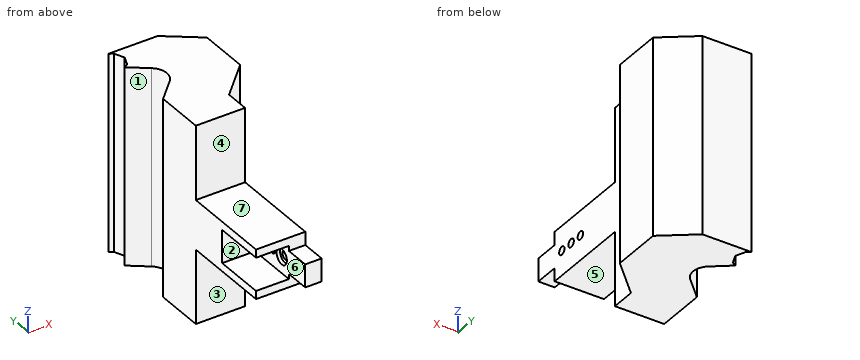
Autodesk Inventor part; units mm, degrees
ref_plane "Work Plane1" through (0, 0, -15) normal (0, 0, 1) x (1, 0, 0)
ref_plane "YZ Plane" through (0, 0, 0) normal (1, 0, 0) x (0, 1, 0)
ref_plane "XZ Plane" through (0, 0, 0) normal (0, 1, 0) x (-1, 0, 0)
sketch "Sketch1" plane through (0, 0, 0) normal (0, 0, 1) x (1, 0, 0)
  line L0 (0, 0) -> (25, 0)
  line L1 (25, 0) -> (25, 40)
  line L2 (25, 40) -> (0, 40)
  line L3 (0, 40) -> (0, 0)
  dimension "d1" = 25
  dimension "d2" = 40
  dimension "d3" = 25
extrude "Extrusion1" add sketch "Sketch1" against normal blind 30
sketch "Sketch2" plane through (25, 0, 0) normal (1, 0, 0) x (0, 0, -1)
  line L0 (0, 0) -> (30, 0)
  circle A0 centre (15, 6.56) radius 2.46
extrude "Extrusion2" cut sketch "Sketch2" against normal blind 30
sketch "Sketch3" plane through (0, 0, 0) normal (-1, 0, 0) x (0, 0, 1)
  line L0 (0, 0) -> (-30, 0)
  line L1 (-25.05, 0) -> (-4.95, 0)
  line L2 (-4.95, 0) -> (-4.95, 33.12)
  line L3 (-4.95, 33.12) -> (-25.05, 33.12)
  line L4 (-25.05, 33.12) -> (-25.05, 0)
  dimension "d11" = 20.1
extrude "Extrusion3" cut sketch "Sketch3" against normal blind 20
sketch "Sketch4" plane through (0, 0, 0) normal (0, -1, 0) x (1, 0, 0)
  line L0 (20, -4.95) -> (20, -25.05)
  line L1 (20, -15) -> (25, -15)
  line L2 (25, 0) -> (25, -30)
  line L3 (20, -8.025) -> (25, -8.025)
  line L4 (25, -8.025) -> (25, -21.975)
  line L5 (25, -21.975) -> (20, -21.975)
  line L6 (20, -21.975) -> (20, -8.025)
  line L7 (20, -8.025) -> (25, -21.975) construction
  line L8 (25, -8.025) -> (20, -21.975) construction
  line L9 (25, -12.54) -> (25, -17.46)
  point P0 (0, 0)
  point P1 (22.5, -15)
  dimension "d14" = 13.95
extrude "Extrusion4" add sketch "Sketch4" along normal blind 15
sketch "Sketch5" plane through (20, 0, 0) normal (-1, 0, 0) x (0, 0, 1)
  circle A0 centre (-15, 6.56) radius 2.46
  circle A1 centre (-15, 6.56) radius 4.7025
  circle A2 centre (-15, 6.56) radius 2.46
  circle A3 centre (-15, 6.56) radius 2.46
  point P0 (0, 0)
  dimension "d17" = 9.405
extrude "Extrusion5" cut sketch "Sketch5" against normal blind 2.1
sketch "Sketch6" plane through (25, 0, 0) normal (1, 0, 0) x (0, 0, -1)
  circle A0 centre (15, 6.56) radius 4.7025
  line L0 (15, 6.56) -> (15, 23.56)
  circle A1 centre (15, 23.56) radius 2.46
  point P0 (0, 0)
  dimension "d20" = 17
  dimension "d21" = 4.92
extrude "Extrusion6" cut sketch "Sketch6" against normal blind 10 contours A1
sketch "Sketch7" plane through (20, 0, 0) normal (-1, 0, 0) x (0, 0, 1)
  circle A0 centre (-15, 23.56) radius 2.46
  circle A1 centre (-15, 23.56) radius 4.7025
  point P0 (0, 0)
  dimension "d24" = 9.405
extrude "Extrusion7" cut sketch "Sketch7" against normal blind 2.1
sketch "Sketch9" plane through (25, 0, 0) normal (1, 0, 0) x (0, 0, -1)
  circle A0 centre (15, 6.56) radius 2.46
  circle A1 centre (15, 6.56) radius 2.46
  circle A2 centre (15, 23.56) radius 2.46
  circle A3 centre (15, 23.56) radius 2.46
  line L0 (30, 40) -> (30, 0)
  line L1 (30, 0) -> (30, 40)
  line L2 (30, 40) -> (0, 40)
  line L3 (0, 40) -> (0, 0)
  line L4 (0, 0) -> (8.025, 0)
  line L5 (21.975, 0) -> (21.975, -15)
  line L6 (21.975, -15) -> (8.025, -15)
  line L7 (8.025, -15) -> (8.025, 0)
  line L8 (0, 0) -> (8.025, 0)
  line L9 (21.975, 0) -> (30, 0)
extrude "Extrusion8" add sketch "Sketch9" along normal blind 5
sketch "Sketch10" plane through (0, 40, 0) normal (0, 1, 0) x (1, 0, 0)
  line L0 (0, 30) -> (30, 30)
  line L1 (30, 0) -> (0, 0)
  line L2 (0, 30) -> (30, 30)
  line L3 (30, 30) -> (30, 0)
  line L4 (30, 0) -> (0, 0)
  line L5 (0, 0) -> (0, 30)
extrude "Extrusion9" add sketch "Sketch10" along normal blind 30
sketch "Sketch12" plane through (30, 0, 0) normal (1, 0, 0) x (0, 0, -1)
  circle A0 centre (15, 6.56) radius 2.46
  line L0 (15, 6.56) -> (15, 15.06)
  circle A1 centre (15, 15.06) radius 2.525
  point P0 (0, 0)
  dimension "d31" = 8.5
  dimension "d33" = 5.05
extrude "Extrusion10" cut sketch "Sketch12" against normal blind 30 contours A1
sketch "Sketch15" plane through (0, 0, -25.05) normal (-1, 0, 0) x (0, 0, 1)
  line L0 (0, 33.12) -> (20.1, 33.12)
  line L1 (20.1, 33.12) -> (20.1, 0)
  line L2 (0, 33.12) -> (20.1, 33.12)
  line L3 (20.1, 33.12) -> (20.1, 31.1)
  line L4 (20.1, 31.1) -> (0, 31.1)
  line L5 (0, 31.1) -> (0, 33.12)
  point P0 (25.05, 0)
  dimension "d57" = 2.02
extrude "Extrusion13" add sketch "Sketch15" against normal blind 20
sketch "Sketch17" plane through (0, 0, 0) normal (0, 0, 1) x (1, 0, 0)
  line L0 (0, 70) -> (30, 70)
  line L1 (30, 70) -> (50.0622, 90.0622)
  line L2 (30, 70) -> (80, 70) construction
  line L3 (11.9522, 97.2454) -> (0, 85.2932)
  line L4 (0, 70) -> (0, 85.2932)
  line L5 (0, 70) -> (0, 0)
  line L6 (0, 70) -> (30, 70)
  line L7 (10.923, 112.2849) -> (0, 120.567)
  line L8 (2.5, 134.067) -> (0, 135.567)
  line L9 (2.5, 134.067) -> (5, 128.067)
  line L10 (2.5, 122.067) -> (0, 120.567)
  line L11 (2.5, 122.067) -> (5, 128.067)
  line L12 (50.0622, 105.3553) -> (50.0622, 120.567)
  line L13 (50.0622, 105.3553) -> (50.0622, 90.0622)
  line L14 (0, 135.567) -> (30, 135.567)
  line L15 (30, 135.567) -> (50.0622, 120.567)
  arc A0 (11.9522, 97.2454) -> (10.923, 112.2849) centre (4.8811, 104.3165) ccw
  dimension "d61" = 45
  dimension "d62" = 32.0271
  dimension "d71" = 30
  dimension "d72" = 10
extrude "Extrusion14" add sketch "Sketch17" against normal blind 30
sketch "Sketch19" plane through (0, 0, 0) normal (0, 0, 1) x (1, 0, 0)
  line L0 (30, 0) -> (30, 70)
  line L1 (30, 70) -> (50.0622, 90.0622)
  line L2 (30, 70) -> (50.0622, 90.0622)
  line L3 (50.0622, 120.567) -> (50.0622, 90.0622)
  line L4 (50.0622, 90.0622) -> (50.0622, 120.567)
  line L5 (30, 135.567) -> (50.0622, 120.567)
  line L6 (50.0622, 120.567) -> (30, 135.567)
  line L7 (0, 135.567) -> (30, 135.567)
  line L8 (30, 135.567) -> (0, 135.567)
  line L9 (5, 128.067) -> (2.5, 134.067)
  line L10 (0, 135.567) -> (2.5, 134.067)
  line L11 (2.5, 134.067) -> (5, 128.067)
  line L12 (2.5, 122.067) -> (5, 128.067)
  line L13 (5, 128.067) -> (2.5, 122.067)
  line L14 (0, 120.567) -> (2.5, 122.067)
  line L15 (2.5, 122.067) -> (0, 120.567)
  line L16 (10.923, 112.2849) -> (0, 120.567)
  line L17 (0, 120.567) -> (10.923, 112.2849)
  line L18 (11.9522, 97.2454) -> (0, 85.2932)
  line L19 (11.9522, 97.2454) -> (0, 85.2932)
  line L20 (0, 85.2932) -> (0, 55.2932)
  line L21 (0, 0) -> (0, 85.2932)
  line L22 (0, 55.2932) -> (30, 55.2932)
  line L23 (30, 55.2932) -> (30, 70)
  arc A0 (11.9522, 97.2454) -> (10.923, 112.2849) centre (4.8811, 104.3165) ccw
  dimension "d75" = 30
  dimension "d76" = 30
extrude "Extrusion15" add sketch "Sketch19" along normal blind 45
ref_plane "Work Plane1" through (0, 0, -15) normal (0, 0, 1) x (1, 0, 0)
mirror "Mirror1" about plane through (0, 0, -15) normal (0, 0, 1) of "Extrusion15"
properties part number "rec_c_12mm_x_120mm"
Here's how the part is built. I have some questions about the finished solid (model axes, mm). Face numbers are marked on the shaded views. A direction names the side the tool comes from. Round coordinates to 2 decimals unless told otherwise and drop trailing zeros. Order: outer loops, then holes, each group sorted by start corner. A loop starts at its lowest first (then second) coordinate and runs counter-clockwise, first axis right, second up. Notation, with made-up numbers: (38, -18.5) -> (94, -18.5) arc R21 ccw to (94, 13.5) -> close; hole circle Ø3 at (-35.5, -35). An arc over 180 degrees is marked (long way). Return JSON: item names as keys, results as strings.
Q1. Which directions (+Z, -Z, +X, -X, +Y, -Y) give clear straight access to the entire face, cutting with the end or side of a thin tool? Please do the marked faces 1, 2 and 3.
Filled sheet:
{"face 1": "+Z, -Z, -X", "face 2": "-X, -Y", "face 3": "-Z, +X, -X, -Y"}
Q2. I need wall thicknesses on line 1 along Y through (x, z) = (21.5, -15) (1 decimal); line 2 along Y through (x, z) = (25.25, -15) (3 decimals); line 3 along Z through (x, y) = (11, 8). Which ranges of each line are inside material? Lowest first, please. Write a range as from..to.
Filled sheet:
{"line 1": "y = -15..1.9, 11.3..12.5, 17.6..18.9, 28.3..135.6", "line 2": "y = -15..4.1, 9.02..12.535, 17.585..21.1, 26.02..135.567", "line 3": "z = -30..-25.05, -4.95..0"}
Q3. If we section it at C-C on z = 14: List the corners of the cut face in (x, y) for me.
Filled sheet:
{"outline": "(0, 55.29) -> (30, 55.29) -> (30, 70) -> (50.06, 90.06) -> (50.06, 120.57) -> (30, 135.57) -> (0, 135.57) -> (2.5, 134.07) -> (5, 128.07) -> (2.5, 122.07) -> (0, 120.57) -> (10.92, 112.28) arc R10 cw to (11.95, 97.25) -> (0, 85.29) -> close"}
Q4. If we section it at D-D on x = 8: List the corners of the cut face in (y, z) for me, plus the area to 3 significant figures.
Filled sheet:
{"outline": "(0, -30) -> (55.29, -30) -> (55.29, -75) -> (93.29, -75) -> (93.29, 45) -> (55.29, 45) -> (55.29, 0) -> (0, 0) -> (0, -4.95) -> (31.1, -4.95) -> (31.1, -25.05) -> (0, -25.05) -> close; (114.5, -75) -> (135.57, -75) -> (135.57, 45) -> (114.5, 45) -> close", "area": "8,120 mm^2"}
Q5. For pin 1 Ø6 at (x, z) = (9, -13) entering from -Y; pin 2 Ø11 at (y, z) = (6.56, -15) entering from -X; pin 3 Ø11 at (y, z) = (23.56, -15) entering from +X; pin 4 Ø6 at (x, y) = (8, 93.5) entering from -Z, each with a flat end and sliding along its axis, tell me the tip position at first contact or that it passes through.
Filled sheet:
{"pin 1": "stops at y = 31.1", "pin 2": "stops at x = 20", "pin 3": "stops at x = 30", "pin 4": "stops at z = -75"}
Q6. If we section it at A-A on x = 27: List the corners of the cut face in (y, z) for me (3 decimals).
Filled sheet:
{"outline": "(-15, -21.975) -> (0, -21.975) -> (0, -30) -> (55.293, -30) -> (55.293, -75) -> (135.567, -75) -> (135.567, 45) -> (55.293, 45) -> (55.293, 0) -> (0, 0) -> (0, -8.025) -> (-15, -8.025) -> close; hole circle Ø4.92 at (6.56, -15); hole circle Ø5.05 at (15.06, -15); hole circle Ø4.92 at (23.56, -15)"}
Q7. If we mould it in two halves opening along Z, with no side actions, what happens to the marked faces 4, 5, 6 and 7? For each: released by +Z, released by -Z, zero draft, split by the parting line, or undercut.
Filled sheet:
{"face 4": "zero draft", "face 5": "released by -Z", "face 6": "undercut", "face 7": "released by +Z"}
Q8. If we section it at B-B on y = 6.56: List the corners of the cut face in (x, z) for me.
Filled sheet:
{"outline": "(0, -30) -> (30, -30) -> (30, -17.46) -> (22.1, -17.46) -> (22.1, -19.7) -> (20, -19.7) -> (20, -25.05) -> (0, -25.05) -> close; (0, -4.95) -> (20, -4.95) -> (20, -10.3) -> (22.1, -10.3) -> (22.1, -12.54) -> (30, -12.54) -> (30, 0) -> (0, 0) -> close"}
